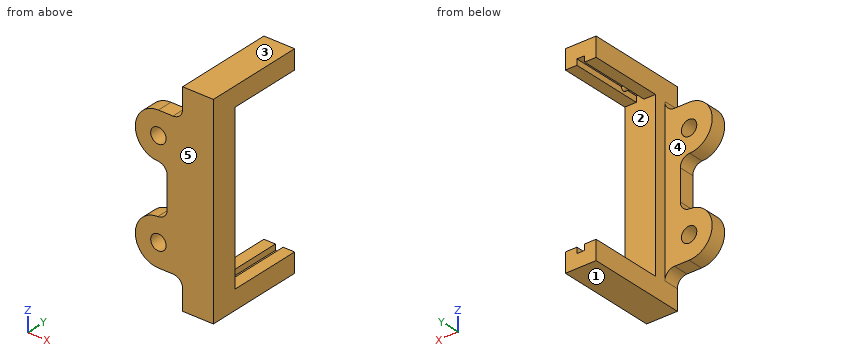
```python
from build123d import *

# Parameters (mm, degrees)
SKETCH1_R           = 2
BOSS_EXTRUDE1_DEPTH = 4
SKETCH1_3_W         = 8
SKETCH1_3_H         = 18.5
SKETCH1_3_H_2       = 7.8
BOSS_EXTRUDE2_DEPTH = 7
BOSS_EXTRUDE3_DEPTH = 22
BOSS_EXTRUDE4_DEPTH = 2
FILLET1_R           = 2.5


with BuildPart() as part:
    # Sketch1 → Boss-Extrude1 (new body)
    with BuildSketch(Plane(origin=(0, 0, 0), x_dir=(1, 0, 0), z_dir=(0, 1, 0))):
        with BuildLine():
            Line((28.947984737, 18.5), (22.647984737, 18.5))
            ThreePointArc((22.647984737, 18.5), (16.647984737, 12.5), (22.647984737, 6.5))
            Line((22.647984737, 6.5), (24.947984737, 6.5))
            Line((24.947984737, 6.5), (24.947984737, -6.5))
            Line((24.947984737, -6.5), (22.647984737, -6.5))
            ThreePointArc((22.647984737, -6.5), (16.647984737, -12.5), (22.647984737, -18.5))
            Line((22.647984737, -18.5), (28.947984737, -18.5))
            Line((28.947984737, -18.5), (28.947984737, 18.5))
        make_face()
        with Locations((22.647984737, 12.5)):
            Circle(SKETCH1_R, mode=Mode.SUBTRACT)
        with Locations((22.647984737, -12.5)):
            Circle(SKETCH1_R, mode=Mode.SUBTRACT)
    extrude(amount=BOSS_EXTRUDE1_DEPTH)

    # Sketch1<3> → Boss-Extrude2 (add)
    with BuildSketch(Plane(origin=(0, 0, 0), x_dir=(1, 0, 0), z_dir=(0, 1, 0))):
        with Locations((32.947984737, 9.25)):
            Rectangle(SKETCH1_3_W, SKETCH1_3_H)
        with Locations((32.947984737, -9.25)):
            Rectangle(SKETCH1_3_W, SKETCH1_3_H)
        with Locations((32.947984737, 22.4)):
            Rectangle(SKETCH1_3_W, SKETCH1_3_H_2)
        with Locations((32.947984737, -22.4)):
            Rectangle(SKETCH1_3_W, SKETCH1_3_H_2)
    extrude(amount=BOSS_EXTRUDE2_DEPTH)

    # Sketch5 → Boss-Extrude3 (add)
    with BuildSketch(Plane(origin=(0, 4, 0), x_dir=(1, 0, 0), z_dir=(0, 1, 0))):
        Polygon((31.947984737, 21.3), (31.947984737, 22.8), (32.947984737, 22.8), (32.947984737, 26.3), (28.947984737, 26.3), (28.947984737, 21.3), align=None)
        Polygon((32.947984737, 26.3), (32.947984737, 22.8), (33.947984737, 22.8), (33.947984737, 21.3), (36.947984737, 21.3), (36.947984737, 26.3), align=None)
        Polygon((36.947984737, -26.3), (36.947984737, -21.3), (33.947984737, -21.3), (33.947984737, -22.8), (32.947984737, -22.8), (32.947984737, -26.3), align=None)
        Polygon((28.947984737, -26.3), (32.947984737, -26.3), (32.947984737, -22.8), (31.947984737, -22.8), (31.947984737, -21.3), (28.947984737, -21.3), align=None)
    extrude(amount=BOSS_EXTRUDE3_DEPTH)

    # Sketch6 → Boss-Extrude4 (add)
    with BuildSketch(Plane(origin=(31.947984737, 0, 0), x_dir=(0, 0, -1), z_dir=(1, 0, 0))):
        with BuildLine():
            Line((22.8, 10.25), (22.8, 11.75))
            ThreePointArc((22.8, 11.75), (22.05, 11), (22.8, 10.25))
        make_face()
        with BuildLine():
            ThreePointArc((-22.8, 11.75), (-22.05, 11), (-22.8, 10.25))
            Line((-22.8, 10.25), (-22.8, 11.75))
        make_face()
    extrude(amount=BOSS_EXTRUDE4_DEPTH)

    # Fillet1
    fillet1_edges = [part.edges().sort_by_distance(p)[0] for p in [
        (28.947984737, 2, 18.5),
        (24.947984737, 2, 6.5),
        (24.947984737, 2, -6.5),
        (28.947984737, 2, -18.5),
    ]]
    fillet(fillet1_edges, radius=FILLET1_R)


solid = part.part
```
CAD build for the part. Positions are in the model's coordinates, mm. Face numbers are marked on the shaded views. A direction names the side the tool comes from. Round coordinates to 2 decimals unless told otherwise and drop trailing zeros. Write each loop counter-clockwise with the first axis right and the second up, starting at its lowest first coordinate (ties: lowest second). Pieces come first, ordered by that corner, then holes. Notation, with made-up numbers: (79.5, 88) -> (116.5, 88) arc R24 cw to (116.5, 125) -> close; hole circle Ø10 at (-23, -12.5). An arc over 180 degrees is marked (long way). Answer in a Markdown table with one row per item. Add a question column.
Item 1: Mould opens along Z. For the marked faces 1, 2 and 3 say: pulls with the +Z half, pulls with the -Z half, needs draft (parallel to the pull), parting line crosses it, or undercut.
Item 2: Drop flat-ended pins along their axis: pin 1 Ø3 at (x, y) = (24.5, 3) entering from -Z; pin 2 Ø10 at (x, z) = (25, -1) entering from +Y; pin 3 Ø4 at (x, y) = (24, 3) entering from +Z; pin 4 Ø3 at (x, z) = (22.65, 12.5) entering from -Y. Give the stop position or say it passes through.
Item 3: Drill centre lines: line 1 (X direction, y = 1.95, z = 12.5); line 2 (Z direction, x = 34, y = 22.5); line 3 (Y direction, x = 31.5, z = -12). Where is each one in solid material? Low to high. Write a range as from..to.
Item 4: Saw through at D-D, the plane x = 29.5. Write the cut outline in (y, z), then the cut area to 3 significant figures.
Item 5: Saw through at A-A, the plane z = -12.5. Write the cut outline in (x, y).
Item 6: Which spindle directions (+Z, -Z, +X, -X, +Y, -Y) get a long thin tool onto all of the face, cutting with end or side? Do the marked faces 4 and 5. Say none if no direction does.
Item 7: Saw through at C-C, the plane x = 18.25. Write the cut outline in (y, z), then the cut area to 3 significant figures.
Item 8: Saw through at B-B, the plane y = 11. Write the cut outline in (x, z).
Findings below:
| question | item | result |
|---|---|---|
| 1 | face 1 | pulls with the -Z half |
| 1 | face 2 | undercut |
| 1 | face 3 | pulls with the +Z half |
| 2 | pin 1 | stops at z = -18.5 |
| 2 | pin 2 | stops at y = 7 |
| 2 | pin 3 | stops at z = 18.5 |
| 2 | pin 4 | passes through |
| 3 | line 1 | x = 16.65..20.65, 24.65..36.95 |
| 3 | line 2 | z = -26.3..-21.3, 21.3..26.3 |
| 3 | line 3 | y = 0..7 |
| 4 | outline | (0, -26.3) -> (26, -26.3) -> (26, -21.3) -> (7, -21.3) -> (7, 21.3) -> (26, 21.3) -> (26, 26.3) -> (0, 26.3) -> close |
| 4 | area | 558 mm^2 |
| 5 | outline | (16.65, 0) -> (20.65, 0) -> (20.65, 4) -> (16.65, 4) -> close; (24.65, 0) -> (36.95, 0) -> (36.95, 7) -> (28.95, 7) -> (28.95, 4) -> (24.65, 4) -> close |
| 6 | face 4 | +Z, -Z, -X, +Y |
| 6 | face 5 | +Z, -Z, +X, -X, -Y |
| 7 | outline | (0, -16.58) -> (4, -16.58) -> (4, -8.42) -> (0, -8.42) -> close; (0, 8.42) -> (4, 8.42) -> (4, 16.58) -> (0, 16.58) -> close |
| 7 | area | 65.3 mm^2 |
| 8 | outline | (28.95, -26.3) -> (36.95, -26.3) -> (36.95, -21.3) -> (33.95, -21.3) -> (33.95, -22.05) -> (31.95, -22.05) -> (31.95, -21.3) -> (28.95, -21.3) -> close; (28.95, 21.3) -> (31.95, 21.3) -> (31.95, 22.05) -> (33.95, 22.05) -> (33.95, 21.3) -> (36.95, 21.3) -> (36.95, 26.3) -> (28.95, 26.3) -> close |
